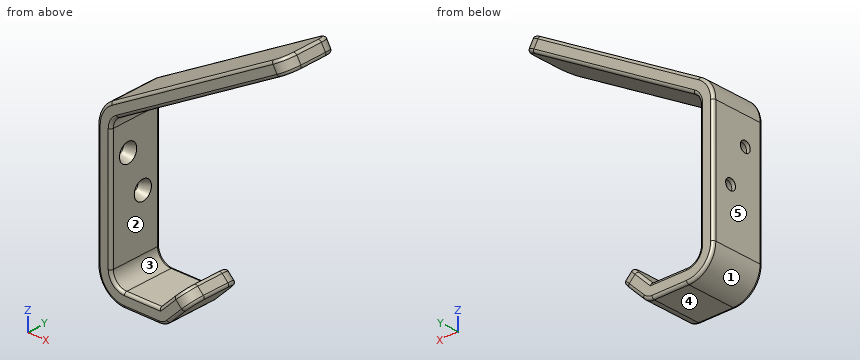
from build123d import *

# Parameters (mm, degrees)
F1_DEPTH        = 20
F2_R            = 10
F3_R            = 5
F4_R            = 5
F5_R            = 10
F6_R            = 5
F7_R            = 5
F8_R            = 5
F9_R            = 5
F10_R           = 5
F11_R           = 1
F12_R           = 1
F13_R           = 1
F15_D           = 4
F15_CSINK_D     = 7
F15_CSINK_ANGLE = 45
F16_D           = 4
F16_CSINK_D     = 7
F16_CSINK_ANGLE = 45


with BuildPart() as f1:
    # F0 (on Front) → F1 (new body)
    with BuildSketch(Plane.XZ):
        Polygon((-14.583103, 18.615519), (-14.583103, -41.384481), (10.416897, -41.384481), (21.023498, -30.777879), (17.487964, -27.242345), (8.544218, -36.186092), (-9.583103, -36.26743), (-9.583103, 15.728768), (57.198929, 54.285392), (54.698929, 58.615519), align=None)
    extrude(amount=F1_DEPTH)

    # F2
    f2_edges = [f1.edges().sort_by_distance(p)[0] for p in [
        (-14.583103, -10, -41.384481),
    ]]
    fillet(f2_edges, radius=F2_R)

    # F3
    f3_edges = [f1.edges().sort_by_distance(p)[0] for p in [
        (-9.583103, -10, -36.26743),
    ]]
    fillet(f3_edges, radius=F3_R)

    # F4
    f4_edges = [f1.edges().sort_by_distance(p)[0] for p in [
        (-9.583103, -10, 15.728768),
    ]]
    fillet(f4_edges, radius=F4_R)

    # F5
    f5_edges = [f1.edges().sort_by_distance(p)[0] for p in [
        (-14.583103, -10, 18.615519),
    ]]
    fillet(f5_edges, radius=F5_R)

    # F6
    f6_edges = [f1.edges().sort_by_distance(p)[0] for p in [
        (19.255731, 0, -29.010112),
    ]]
    fillet(f6_edges, radius=F6_R)

    # F7
    f7_edges = [f1.edges().sort_by_distance(p)[0] for p in [
        (19.255731, -20, -29.010112),
    ]]
    fillet(f7_edges, radius=F7_R)

    # F8
    f8_edges = [f1.edges().sort_by_distance(p)[0] for p in [
        (55.948929, 0, 56.450456),
    ]]
    fillet(f8_edges, radius=F8_R)

    # F9
    f9_edges = [f1.edges().sort_by_distance(p)[0] for p in [
        (55.948929, -20, 56.450456),
    ]]
    fillet(f9_edges, radius=F9_R)

    # F10
    f10_edges = [f1.edges().sort_by_distance(p)[0] for p in [
        (10.416897, -10, -41.384481),
    ]]
    fillet(f10_edges, radius=F10_R)

    # F11
    f11_edges = [f1.edges().sort_by_distance(p)[0] for p in [
        (22.892849, -20, 34.478768),
    ]]
    fillet(f11_edges, radius=F11_R)

    # F12
    f12_edges = [f1.edges().sort_by_distance(p)[0] for p in [
        (20.392849, -20, 38.808895),
    ]]
    fillet(f12_edges, radius=F12_R)

    # F13
    f13_edges = [f1.edges().sort_by_distance(p)[0] for p in [
        (11.248324, -20, -33.481985),
    ]]
    fillet(f13_edges, radius=F13_R)

    # F15 (through all)
    with Locations(Plane.YZ.offset(-9.583103)):
        with Locations((-7, -11.244944)):
            CounterSinkHole(F15_D / 2, F15_CSINK_D / 2, counter_sink_angle=F15_CSINK_ANGLE)

    # F16 (through all)
    with Locations(Plane.YZ.offset(-9.583103)):
        with Locations((-13, 2.842016)):
            CounterSinkHole(F16_D / 2, F16_CSINK_D / 2, counter_sink_angle=F16_CSINK_ANGLE)


solid = f1.part
Here's how the part is built. I have some questions about the finished solid (model axes, mm). Face numbers are marked on the shaded views. A direction names the side the tool comes from. Give positions to 0.01 mm unless a question says otherwise; leave off trailing zeros. Loops run counter-clockwise (first coordinate to the right, second up) from the corner with the lowest first, then second, coordinate; pieces in that order, holes last. Notation, with made-up numbers: (49, 76.25) -> (102, 76.25) arc R30 ccw to (102, 101.25) -> close; hole circle Ø6 at (-0.5, -37). An arc over 180 degrees is marked (long way). Answer as a JSON object with one key per item and string values. Group by question number.
Item 1: Will these pins go through, and if not, where does the flat tip stop? pin 1 (4 mm diameter, centred on x = 17.5, y = -4, fed in from -Z); pin 2 (1 mm diameter, centred on x = 16.5, z = -28.5, fed in from -Y); pin 3 (5.5 mm diameter, centred on y = -7.5, z = -17.5, fed in from +X); pin 4 (3 mm diameter, centred on y = -7, z = -11.24, fed in from +X).
Item 2: Imagine slicing it at B-B on z = -20.5. Write out the boundary of the cut face in (x, y).
Item 3: Thinking about a two-plate mould opening in X: for the marked faces 3, 4 and 5, which applies, pulls with the +X half, pulls with the -X half, needs draft (parallel to the pull), parting line crosses it, or undercut?
Item 4: I need wall thicknesses on L1, parallel to X at y = -4.5, z = -4; L2, parallel to Z at x = 33.5, y = -5; L3, parallel to Z at x = -5.5, y = -9. Which ranges of each line are inside material? Lowest first, please.
Item 5: On a 3-axis mill with a long thin cutter (end or side, diameter ignored), from which of +Z, -Z, +X, -X, +Y, -Y can I reach the whole of each face in a straight line? I mean the marked faces 1 and 2. Say none if no direction works.
Item 6: Imagine slicing it at A-A on y = -7. Write out the boundary of the cut face in (x, z), then the cut area to 3 significant figures.
Answer list:
{
 "1": {"pin 1": "stops at z = -36.3", "pin 2": "stops at y = -18.82", "pin 3": "stops at x = -9.58", "pin 4": "passes through"},
 "2": {"outline": "(-14.58, -19) arc R1 ccw to (-13.58, -20) -> (-10.58, -20) arc R1 ccw to (-9.58, -19) -> (-9.58, -1) arc R1 ccw to (-10.58, 0) -> (-13.58, 0) arc R1 ccw to (-14.58, -1) -> close"},
 "3": {"face 3": "undercut", "face 4": "needs draft", "face 5": "pulls with the -X half"},
 "4": {"L1": "x = -14.58 to -9.58", "L2": "z = 40.6 to 46.38", "L3": "z = -41.34 to -36.16, 18.09 to 23.86"},
 "5": {"face 1": "-Z, -X, +Y, -Y", "face 2": "+Y, -Y"},
 "6": {"outline": "(-14.58, -31.38) arc R10 ccw to (-4.58, -41.38) -> (8.35, -41.38) arc R5 ccw to (11.88, -39.92) -> (20.32, -31.48) arc R1 ccw to (20.32, -30.07) -> (18.2, -27.95) arc R1 ccw to (16.78, -27.95) -> (8.54, -36.19) -> (-4.56, -36.24) arc R5 cw to (-9.58, -31.24) -> (-9.58, -14.74) -> (-13.2, -13.24) -> (-14.58, -13.24) -> close; (-14.58, -9.24) -> (-13.2, -9.24) -> (-9.58, -7.74) -> (-9.58, 12.84) arc R5 cw to (-7.08, 17.17) -> (56.33, 53.79) arc R1 ccw to (56.7, 55.15) -> (55.2, 57.75) arc R1 ccw to (53.83, 58.12) -> (-9.58, 21.5) arc R10 ccw to (-14.58, 12.84) -> close", "area": "806 mm2"}
}
